Geometry check sheet. Reference: the model listing, model coordinates, mm. Face numbers are marked on the shaded views. A direction names the side the tool comes from. Round coordinates to 2 decimals unless told otherwise and drop trailing zeros. Write each loop counter-clockwise with the first axis right and the second up, starting at its lowest first coordinate (ties: lowest second). Pieces come first, ordered by that corner, then holes. Notation, with made-up numbers: M 13,20 L 18,20 A8 cw 18,33 Z; hole C 62.5,-22.75 d1. An arc over 180 degrees is marked long. Use a Markdown table: item, result.
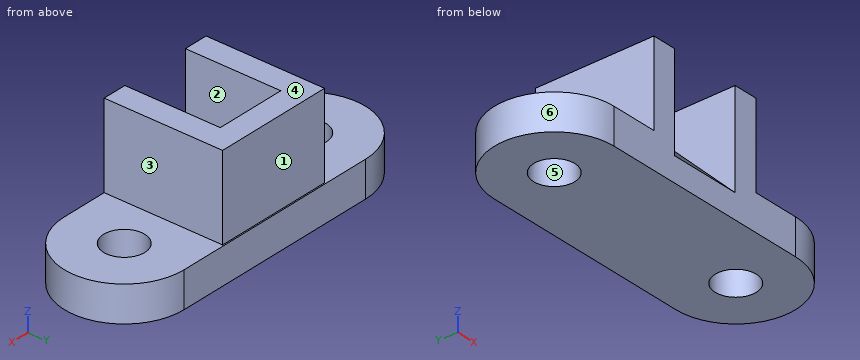
Autodesk Inventor part; units mm, degrees
ref_plane "Work Plane1" through (0, 0, 0) normal (0, 0, 1) x (1, 0, 0)
ref_plane "Work Plane2" through (0, 0, 0) normal (0, 0, 1) x (1, 0, 0)
ref_plane "YZ Plane" through (0, 0, 0) normal (1, 0, 0) x (0, 1, 0)
sketch "Sketch1" plane through (0, 0, 0) normal (0, 0, 1) x (1, 0, 0)
  point P0 (0, 0)
sketch "Sketch2" plane through (0, 0, 0) normal (0, 0, 1) x (1, 0, 0)
  line L0 (-53.7332, 0) -> (60.2668, 0) construction
  line L1 (-53.7332, -32) -> (60.2668, -32)
  line L2 (60.2668, 32) -> (-53.7332, 32)
  arc A0 (-53.7332, 32) -> (-53.7332, -32) centre (-53.7332, 0) ccw
  arc A1 (60.2668, -32) -> (60.2668, 32) centre (60.2668, 0) ccw
  point P0 (0, 0)
  point P1 (3.2668, 0)
  dimension "d0" = 32
  dimension "d1" = 32
  dimension "d2" = 114
extrude "Extrusion1" add sketch "Sketch2" against normal blind 19
ref_plane "Work Plane1" through (0, 0, 0) normal (0, 0, 1) x (1, 0, 0)
sketch "Sketch3" plane through (0, 0, 0) normal (0, 0, 1) x (1, 0, 0)
  arc A0 (60.2668, -32) -> (60.2668, 32) centre (60.2668, 0) ccw
  line L0 (60.2668, -32) -> (-53.7332, -32)
  line L1 (-28.7332, -32) -> (-28.7332, 31.3001)
  line L2 (35.2668, -32) -> (35.2668, 31.3001)
  line L3 (-53.7332, -32) -> (60.2668, -32)
  line L4 (-15.7332, -32) -> (-15.7332, 19)
  line L5 (22.2668, 19) -> (22.2668, -32)
  line L6 (-15.7332, 19) -> (22.2668, 19)
  line L7 (-28.7332, 31.3001) -> (35.2668, 31.3001)
  line L8 (-53.7332, 32) -> (60.2668, 32)
  point P0 (0, 0)
  point P1 (-54.8329, -31.8056)
  point P2 (3.2668, -32)
  point P3 (3.2668, -32)
  point P4 (3.2668, -32)
  point P5 (-15.7332, 32)
  point P6 (20.2211, 31.3001)
  point P7 (3.2668, -32)
  point P8 (3.2668, -32)
  point P9 (22.2668, -32)
  point P10 (3.2668, -32)
  point P11 (3.2668, -32)
  dimension "d6" = 58.0997
  dimension "d7" = 64
  dimension "d12" = 51
  dimension "d17" = 38
  dimension "d18" = 19
  dimension "d19" = 19
extrude "Extrusion2" add sketch "Sketch3" along normal blind 45 contours L0 L5 L6 L4 L1 L7 L2
ref_plane "Work Plane2" through (0, 0, 0) normal (0, 0, 1) x (1, 0, 0)
sketch "Sketch5" plane through (-53.7332, -32, -19) normal (0, -1, 0) x (1, 0, 0)
  line L0 (38, 19) -> (76, 19)
  line L1 (38, 19) -> (76, 19)
  line L2 (76, 19) -> (76, 13)
  line L3 (76, 13) -> (38, 13)
  line L4 (38, 13) -> (38, 19)
  point P0 (53.7332, 19)
  dimension "d16" = 38
  dimension "d20" = 6
extrude "Extrusion3" cut sketch "Sketch5" against normal blind 51
sketch "Sketch6" plane through (-15.7332, -32, 45) normal (1, 0, 0) x (0, 0, -1)
  line L0 (0, 51) -> (51, 51)
  line L1 (51, 51) -> (51, 0)
  line L2 (51, 0) -> (0, 51)
  point P0 (45, 32)
extrude "Extrusion4" add sketch "Sketch6" along normal blind 51
sketch "Sketch7" plane through (0, 0, 0) normal (0, 0, 1) x (1, 0, 0)
  line L0 (-28.7332, -32) -> (-28.7332, 31.3001)
  line L1 (-28.7332, 31.3001) -> (35.2668, 31.3001)
  line L2 (35.2668, 31.3001) -> (35.2668, -32)
  line L3 (35.2668, -32) -> (60.2668, -32)
  arc A0 (60.2668, -32) -> (60.2668, 32) centre (60.2668, 0) ccw
  line L4 (60.2668, 32) -> (-53.7332, 32)
  arc A1 (-53.7332, 32) -> (-53.7332, -32) centre (-53.7332, 0) ccw
  line L5 (-53.7332, -32) -> (-28.7332, -32)
  circle A2 centre (-53.7332, 0) radius 11
  circle A3 centre (60.2668, 0) radius 11
  point P0 (0, 0)
  dimension "d25" = 22
  dimension "d26" = 22
  dimension "d27" = 114
extrude "Extrusion5" cut sketch "Sketch7" against normal through all contours A2 | A3
properties material "Nylon 6/6"
Item 1: Access from +Z, -Z, +X, -X, +Y, -Y to the whole of each face (thin tool, end or side, straight path). Record for the marked faces 1, 2 and 3.
Outcome:
| item | result |
|---|---|
| face 1 | +Z, +X, -X, +Y |
| face 2 | +Z, -Y |
| face 3 | +Z, +X, +Y, -Y |
Item 2: Mould release check, pull along X, two halves, no side actions. Record for the marked faces 4, 5 and 6: +X half, -X half, draft (parallel to the pull), parting line (faces both ways), or undercut.
Outcome:
| item | result |
|---|---|
| face 4 | draft |
| face 5 | undercut |
| face 6 | -X half |
Item 3: Cross-section at A-A, the plane y = 0. Record the cut outline in (x, z), and give its area (3 significant figures).
Outcome:
| item | result |
|---|---|
| outline | M -85.73,-19 L -64.73,-19 L -64.73,0 L -85.73,0 Z; M -42.73,-19 L 49.27,-19 L 49.27,0 L 35.27,0 L 35.27,45 L 22.27,45 L 22.27,26 L -15.73,26 L -15.73,45 L -28.73,45 L -28.73,0 L -42.73,0 Z; M 71.27,-19 L 92.27,-19 L 92.27,0 L 71.27,0 Z |
| area | 4,700 mm2 |
Item 4: Go/stop test with flat-tipped pins: pin 1 (6 mm diameter, centred on x = -18.5, z = 29, fed in from +Y); pin 2 (15.5 mm diameter, centred on y = -10.5, z = 25, fed in from -X); pin 3 (1 mm diameter, centred on y = -11.5, z = 23.5, fed in from +X). Record where each tip stops, or that it passes through.
Outcome:
| item | result |
|---|---|
| pin 1 | stops at y = 31.3 |
| pin 2 | stops at x = -28.73 |
| pin 3 | stops at x = 35.27 |
Item 5: Material ranges on line 1 along X through (y, z) = (-20.5, 16); line 2 along X through (y, z) = (1, -3); line 3 along X through (y, z) = (-2.5, 21.5), recorded low to high. Write a range as from..to.
Outcome:
| item | result |
|---|---|
| line 1 | x = -28.73..-15.73, 22.27..35.27 |
| line 2 | x = -85.72..-64.69, -42.78..49.31, 71.22..92.25 |
| line 3 | x = -28.73..35.27 |
Item 6: Cross-section at C-C, the plane y = 13. Record the cut outline in (x, z), and give its area (3 significant figures).
Outcome:
| item | result |
|---|---|
| outline | M -82.97,-19 L 89.51,-19 L 89.51,0 L 35.27,0 L 35.27,45 L 22.27,45 L 22.27,39 L -15.73,39 L -15.73,45 L -28.73,45 L -28.73,0 L -82.97,0 Z |
| area | 5,930 mm2 |
Item 7: Cross-section at B-B, the plane z = 26. Record the cut outline in (x, y).
Outcome:
| item | result |
|---|---|
| outline | M -28.73,-32 L -15.73,-32 L -15.73,0 L 22.27,0 L 22.27,-32 L 35.27,-32 L 35.27,31.3 L -28.73,31.3 Z |
Item 8: Cross-section at D-D, the plane z = 39. Record the cut outline in (x, y), and give its area (3 significant figures).
Outcome:
| item | result |
|---|---|
| outline | M -28.73,-32 L -15.73,-32 L -15.73,13 L 22.27,13 L 22.27,-32 L 35.27,-32 L 35.27,31.3 L -28.73,31.3 Z |
| area | 2,340 mm2 |
